```python
from build123d import *

# Parameters (mm, degrees)
BOSS_EXTRUDE1_DEPTH    = 6.35
F_10_CLEARANCE_HOLE1_D = 5.6134
SKETCH2_R              = 6.35
CUT_EXTRUDE1_DEPTH     = 7.35
HOLE1_D                = 3.175
HOLE1_DEPTH            = 31.75
HOLE1_CSINK_D          = 10.16
HOLE1_CSINK_ANGLE      = 82
HOLE1_TIP              = 0.953866233


with BuildPart() as part:
    # Sketch1 → Boss-Extrude1 (new body)
    with BuildSketch(Plane.XY):
        with BuildLine():
            Line((-35.929687435, 42.153790719), (-1.51387348, -351.220762831))
            ThreePointArc((-1.51387348, -351.220762831), (15.815726351, -378.422785743), (48.038169143, -379.829647978))
            Line((48.038169143, -379.829647978), (118.213861049, -347.106185426))
            ThreePointArc((118.213861049, -347.106185426), (132.909364503, -334.218574785), (138.378918258, -315.453385964))
            Line((138.378918258, -315.453385964), (138.378918258, 254.538122714))
            Line((138.378918258, 254.538122714), (-403.099057101, 418.419278389))
            Line((-403.099057101, 418.419278389), (-422.935039487, 352.879420938))
            Line((-422.935039487, 352.879420938), (-398.624090476, 345.521584423))
            Line((-398.624090476, 345.521584423), (-105.026598758, 156.030008008))
            ThreePointArc((-105.026598758, 156.030008008), (-57.378429325, 107.040440177), (-35.929687435, 42.153790719))
        make_face()
    extrude(amount=BOSS_EXTRUDE1_DEPTH)

    # #10 Clearance Hole1 (through all)
    with Locations(Plane(origin=(0, 0, 0), x_dir=(-1, 0, 0), z_dir=(0, 0, -1))):
        with Locations((-24.251683892, -100.351877226), (-24.251683892, -167.026877226), (-75.051683892, -133.689377226), (-29.317369668, -58.274702428), (-25.026257572, -9.227066735), (-62.648775204, -30.647052627)):
            Hole(F_10_CLEARANCE_HOLE1_D / 2)

    # Sketch2 → Cut-Extrude1 (cut, through all)
    with BuildSketch(Plane(origin=(0, 0, 0), x_dir=(-1, 0, 0), z_dir=(0, 0, -1))):
        with Locations((-46.476683892, -133.689377226)):
            Circle(SKETCH2_R)
        with Locations((-36.66056812, -32.920726132)):
            Circle(SKETCH2_R)
    extrude(amount=-CUT_EXTRUDE1_DEPTH, mode=Mode.SUBTRACT)

    # Hole1
    with Locations(Plane(origin=(277.286738577, -215.287141225, 12.7), x_dir=(-0.089959629, 0.995945413, 0), z_dir=(0, 0, 1))):
        with Locations((637.870011036, 553.595098153), (52.960474705, 241.752641108), (47.697836423, 183.489834462), (434.459074831, 134.806234549), (453.103621196, 177.188747915), (499.723341091, 267.496267453), (636.071223534, 609.111420407), (609.449424187, 543.22015483), (559.371199386, 359.303721429), (507.038658285, 229.776136946)):
            CounterSinkHole(HOLE1_D / 2, HOLE1_CSINK_D / 2, depth=HOLE1_DEPTH, counter_sink_angle=HOLE1_CSINK_ANGLE)
            with Locations((0, 0, -(HOLE1_DEPTH + HOLE1_TIP / 2))):  # 118° drill point
                Cone(0, HOLE1_D / 2, HOLE1_TIP, mode=Mode.SUBTRACT)


solid = part.part
```
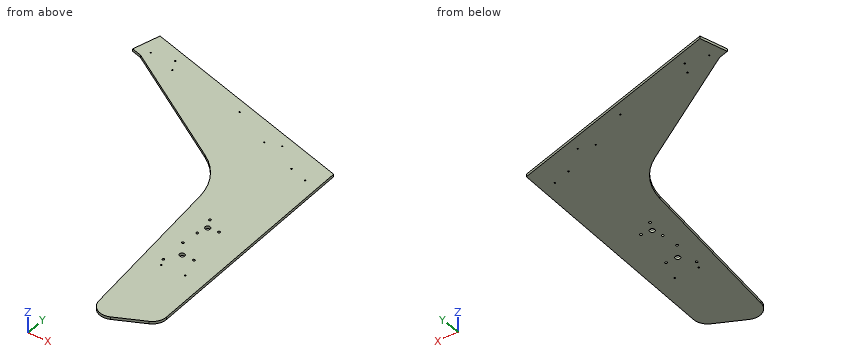
CAD build for the part. Positions are in the model's coordinates, mm. Round coordinates to 2 decimals unless told otherwise and drop trailing zeros. Loops run counter-clockwise (first coordinate to the right, second up) from the corner with the lowest first, then second, coordinate; pieces in that order, holes last. Notation, with made-up numbers: M 86.5,87.25 L 103.5,87.25 A21 cw 103.5,105.25 Z; hole C 61,32.5 d1. An arc over 180 degrees is marked long. Use a Markdown table: item, result. Add a question column.
(1) Cut at C-C (x = -202). Give the cut face in (y, z), and give its area (3 significant figures).
(2) Flat gauge pins, fed straight in: pin 1 (1.9 mm diameter, centred on x = -386.58, y = 363.41, fed in from +Z); pin 2 (1.5 mm diameter, centred on y = -206.5, z = 3.5, fed in from -X). Where does each tip first touch, or does it go through?
(3) Cut at B-B (y = 185). Give the cut face in (x, z).
(4) Drill centre lines: line 1 (Y direction, x = 75, z = 6.25); line 2 (X direction, y = -169.5, z = 4.25); line 3 (X direction, y = -52, z = 2). Where is each one in solid material? Low to high.
(5) Cut at A-A (z = 5). State how many separate pieces and enclosed holes the cut face has, and give its area (3 significant figures).
Geometry says:
| question | item | result |
|---|---|---|
| 1 | outline | M 218.62,0 L 357.56,0 L 357.56,6.35 L 218.62,6.35 Z |
| 1 | area | 882 mm² |
| 2 | pin 1 | passes through |
| 2 | pin 2 | stops at x = -14.24 |
| 3 | outline | M -149.91,0 L 138.38,0 L 138.38,6.35 L -149.91,6.35 Z |
| 4 | line 1 | y = -367.26 to -136.5, -130.88 to 273.72 |
| 4 | line 2 | x = -17.41 to 22.92, 25.58 to 138.38 |
| 4 | line 3 | x = -27.69 to 138.38 |
| 5 | separate pieces | 1 |
| 5 | enclosed holes | 18 |
| 5 | area | 155,000 mm² |
